Autodesk Inventor part; units mm, degrees
ref_plane "YZ Plane" through (0, 0, 0) normal (1, 0, 0) x (0, 1, 0)
ref_plane "XZ Plane" through (0, 0, 0) normal (0, 1, 0) x (-1, 0, 0)
ref_plane "XY Plane" through (0, 0, 0) normal (0, 0, 1) x (1, 0, 0)
sketch "スケッチ1" plane through (0, 0, 0) normal (0, 0, 1) x (1, 0, 0)
  circle A0 centre (0, 0) radius 1
  dimension "d0" = 2
extrude "押し出し1" add sketch "スケッチ1" along normal blind 6
sketch "スケッチ2" plane through (0, 0, 6) normal (0, 0, 1) x (1, 0, 0)
  circle A0 centre (0, 0) radius 1
  circle A1 centre (0, 0) radius 2
  dimension "d3" = 4
extrude "押し出し2" add sketch "スケッチ2" along normal blind 1.35 contours A0 | A1
fillet "フィレット1" radius 1.35 1 edges at (-2, 0, 7.35)
thread "ねじ1"
sketch "スケッチ3" plane through (0, 0, 0) normal (0, 0, -1) x (-1, 0, 0)
  circle A0 centre (0, 0) radius 1
properties part number "SB　M2 6mmなべネジ" material "Steel, Mild"
Here's how the part is built. I have some questions about the finished solid (model axes, mm). A direction names the side the tool comes from. Round coordinates to 2 decimals unless told otherwise and drop trailing zeros. Write each loop counter-clockwise with the first axis right and the second up, starting at its lowest first coordinate (ties: lowest second). Pieces come first, ordered by that corner, then holes.
1. Will these pins go through, and if not, where does the flat tip stop? pin 1 Ø1 at (y, z) = (1, 1.5) entering from +X; pin 2 Ø2 at (y, z) = (1, 5.5) entering from -X; pin 3 Ø1.5 at (y, z) = (-1, 5) entering from +X.
2. For faces 1 (the flat face through (0, 0, 0)), 2 (the cylindrical face through (0, 1, 3)), which set-ups out of +Z, -Z, +X, -X, +Y, -Y let a thin tool reach every point of the face, with its end or its side?
3. Suppose I cut it at A-A (z = 4). List the corners of the cut face in (x, y) for me.
4. I need wall thicknesses on L1, parallel to X at y = 0.05, z = 1.25; L2, parallel to X at y = -0.85, z = 5.5. Which ranges of each line are inside material? Lowest first, please.
Answer sheet:
1. pin 1: stops at x = 0.87
1. pin 2: stops at x = -2
1. pin 3: stops at x = 0.97
2. face 1: -Z, +X, -X, +Y, -Y
2. face 2: -Z
3. outline: circle Ø2 at (0, 0)
4. L1: x = -1 to 1
4. L2: x = -0.53 to 0.53
